Geometry check sheet. Reference: the model listing, model coordinates, mm. A direction names the side the tool comes from. Round coordinates to 2 decimals unless told otherwise and drop trailing zeros. Write each loop counter-clockwise with the first axis right and the second up, starting at its lowest first coordinate (ties: lowest second). Pieces come first, ordered by that corner, then holes. Notation, with made-up numbers: (51, 81) -> (83, 81) arc R22 ccw to (83, 94) -> close; hole circle Ø11 at (70, 16). An arc over 180 degrees is marked (long way). Use a Markdown table: item, result.
```python
from build123d import *

# Parameters (mm, degrees)
PAD_DEPTH            = 25
FILLET_R             = 5
SKETCH001_R          = 2
POCKET_DEPTH         = 12.501
POCKET_DEPTH_BACK    = -12.501
BODY_PLACEMENT_ANGLE = 270


with BuildPart() as part:
    # Sketch → Pad (new body, symmetric)
    with BuildSketch(Plane.XY):
        Polygon((-12.5, 1), (-12.5, -1), (12.5, -1), (12.5, 1), (1, 1), (1, 101), (-1, 101), (-1, 1), align=None)
    extrude(amount=PAD_DEPTH, both=True)

    # Fillet
    fillet_edges = [part.edges().sort_by_distance(p)[0] for p in [
        (-1, 1, 0),
        (1, 1, 0),
    ]]
    fillet(fillet_edges, radius=FILLET_R)

    # Sketch001 → Pocket (cut, two sides)
    with BuildSketch(Plane.YZ) as pocket_sk:
        with Locations((95, 15)):
            Circle(SKETCH001_R)
        with Locations((95, -15)):
            Circle(SKETCH001_R)
    extrude(amount=-POCKET_DEPTH, mode=Mode.SUBTRACT)
    extrude(pocket_sk.sketch, amount=-POCKET_DEPTH_BACK, mode=Mode.SUBTRACT)


with BuildPart() as part_1:
    # Body placement: moved
    add(part.part.rotate(Axis((0, 0, 0), (0, 1, 0)), BODY_PLACEMENT_ANGLE))


solid = part_1.part
```
(1) Thickness scan on line 1 (X direction, y = 95, z = -0.55); line 2 (Y direction, x = 15, z = 0.7); line 3 (Z direction, x = -8.5, y = 65). Record the ranges inside material, lowest first.
A:
| item | result |
|---|---|
| line 1 | x = -25 to -17, -13 to 13, 17 to 25 |
| line 2 | y = -1 to 93, 97 to 101 |
| line 3 | z = -1 to 1 |
(2) Access from +Z, -Z, +X, -X, +Y, -Y to the whole of each face (thin tool, end or side, straight path). Record for faces 1 (the face through (25, 46, 0)), 2 (the face through (0, 54, -1)), 3 (the face through (0, 1, 9)).
A:
| item | result |
|---|---|
| face 1 | +Z, -Z, +X, +Y, -Y |
| face 2 | -Z, +X, -X, +Y |
| face 3 | +Z, +X, -X, +Y |
(3) Section check D-D on x = -3. Record the cut outline in (y, z).
A:
| item | result |
|---|---|
| outline | (-1, -12.5) -> (1, -12.5) -> (1, -6) arc R5 cw to (6, -1) -> (101, -1) -> (101, 1) -> (6, 1) arc R5 cw to (1, 6) -> (1, 12.5) -> (-1, 12.5) -> close |
(4) Section check C-C on z = -8.5. Record the cut outline in (x, y).
A:
| item | result |
|---|---|
| outline | (-25, -1) -> (25, -1) -> (25, 1) -> (-25, 1) -> close |
(5) Section check B-B on y = 95. Record the cut outline in (x, z), plus the area to 3 significant figures.
A:
| item | result |
|---|---|
| outline | (-25, -1) -> (-17, -1) -> (-17, 1) -> (-25, 1) -> close; (-13, -1) -> (13, -1) -> (13, 1) -> (-13, 1) -> close; (17, -1) -> (25, -1) -> (25, 1) -> (17, 1) -> close |
| area | 84.0 mm2 |
(6) Section check A-A on x = -15. Record the cut outline in (y, z).
A:
| item | result |
|---|---|
| outline | (-1, -12.5) -> (1, -12.5) -> (1, -6) arc R5 cw to (6, -1) -> (93, -1) -> (93, 1) -> (6, 1) arc R5 cw to (1, 6) -> (1, 12.5) -> (-1, 12.5) -> close; (97, -1) -> (101, -1) -> (101, 1) -> (97, 1) -> close |
(7) Gauge pin test, flat ends, axial feed: pin 1 Ø2 at (x, y) = (-2, 62) entering from -Z; pin 2 Ø12 at (x, y) = (-12.5, 59) entering from +Z; pin 3 Ø2 at (x, z) = (-4, -8) entering from +Y; pin 4 Ø2.5 at (x, y) = (-15, 95) entering from -Z. Record the tip position at first contact, or that the pin passes through.
A:
| item | result |
|---|---|
| pin 1 | stops at z = -1 |
| pin 2 | stops at z = 1 |
| pin 3 | stops at y = 1 |
| pin 4 | passes through |
